The drawing under review shows one solid part. Ordinate dimensions are in mm from its lowest x, y, z. A direction names the side the tool comes from. Give positions to 0.01 mm unless a question says otherwise; leave off trailing zeros. Order: outer loops, then holes, each group sorted by start corner. A loop starts at its lowest first (then second) coordinate and runs counter-clockwise, first axis right, second up. Notation, with made-up numbers: (60, 79.25) -> (81, 79.25) arc R15 cw to (81, 93.25) -> close; hole circle Ø7 at (-10.75, 79). An arc over 180 degrees is marked (long way). One line per item, written item: value. Start each with the question number.
1) For pin 1 (3 mm diameter, centred on y = 12.5, z = 12.5, fed in from +X); pin 2 (8 mm diameter, centred on x = 81.5, z = 14, fed in from -Y); pin 3 (5 mm diameter, centred on y = 50, z = 25, fed in from -X), all flat-tipped, find the tip position at first contact; note any pin that passes through.
2) Consider section C-C (x = 133.5). State the section outline as (y, z) points, plus the area to 3 significant figures.
3) Tool access review of the marked faces 4, 5, 6, 7 and 8: name each direction out of +Z, -Z, +X, -X, +Y, -Y from which nothing blocks a thin tool from reaching the whole face with its end or side.
4) Consider section B-B (z = 25). State the section outline as (x, y) points, plus the area to 3 significant figures.
5) The part is to be moulded in two halves that separate along X. For the marked faces 1, 2 and 3, say which applies: released by +X, released by -X, zero draft, split by the parting line, or undercut.
6) Wall thickness on line 1 along X through (y, z) = (71.5, 10); line 2 along Y through (x, z) = (135, 25); line 3 along X through (y, z) = (16, 40): over which ranges is each line inside the solid? List them lowest first. Write a range as from..to.
7) Consider section A-A (y = 50). State the section outline as (x, z) points, plus the area to 3 significant figures.
8) Consider section D-D (y = 80.5). State the section outline as (x, z) points, plus the area to 3 significant figures.
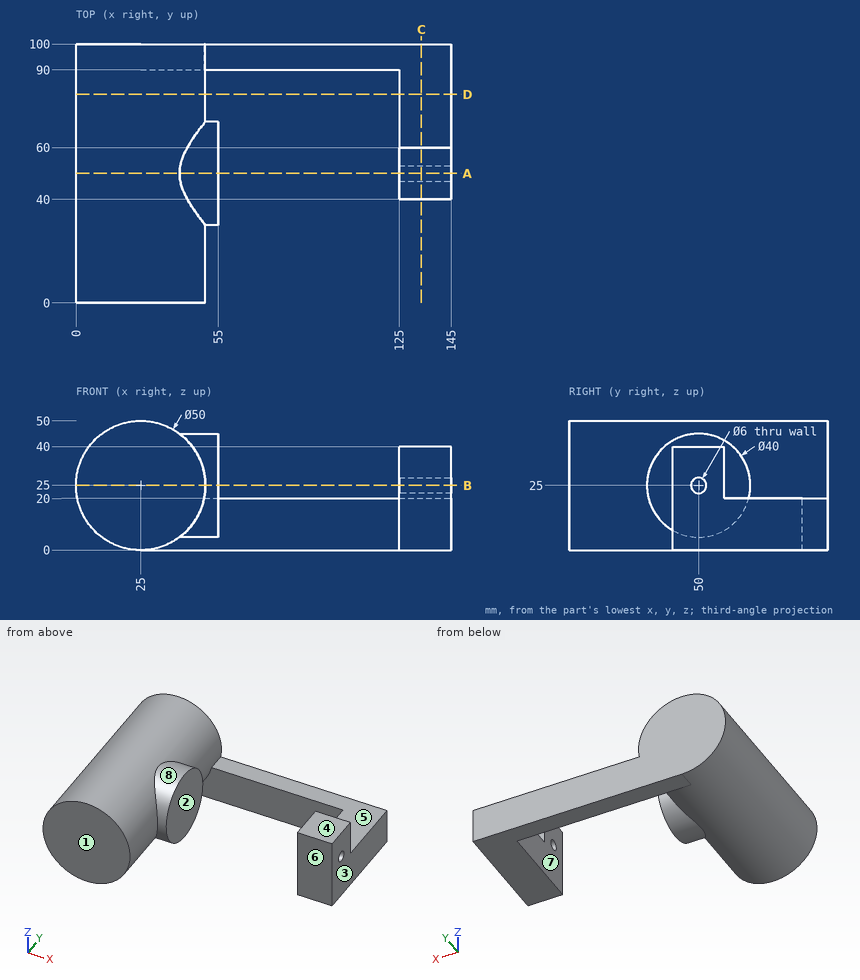
Checked values:
1. pin 1: stops at x = 47.45
1. pin 2: stops at y = 90
1. pin 3: stops at x = 0
2. outline: (40, 0) -> (100, 0) -> (100, 20) -> (60, 20) -> (60, 40) -> (40, 40) -> close; hole circle Ø6 at (50, 25)
2. area: 1,570 mm^2
3. face 4: +Z, +X, +Y, -Y
3. face 5: +Z, +X, +Y
3. face 6: +Z, -Z, +X, -Y
3. face 7: +Z, -Z, -Y
3. face 8: none
4. outline: (0, 0) -> (50, 0) -> (50, 30) -> (55, 30) -> (55, 70) -> (50, 70) -> (50, 100) -> (0, 100) -> close; (125, 40) -> (145, 40) -> (145, 47) -> (125, 47) -> close; (125, 53) -> (145, 53) -> (145, 60) -> (125, 60) -> close
4. area: 5,480 mm^2
5. face 1: zero draft
5. face 2: undercut
5. face 3: released by +X
6. line 1: x = 5..45, 125..145
6. line 2: y = 40..47, 53..60
6. line 3: x = 5..45
7. outline: (40, 5) -> (55, 5) -> (55, 45) -> (40, 45) arc R25 ccw (long way) to start; (125, 0) -> (145, 0) -> (145, 22) -> (125, 22) -> close; (125, 28) -> (145, 28) -> (145, 40) -> (125, 40) -> close
7. area: 2,960 mm^2
8. outline: circle Ø50 at (25, 25); (125, 0) -> (145, 0) -> (145, 20) -> (125, 20) -> close
8. area: 2,360 mm^2
